Source: three-view drawing plus pictorial views. Frame: mm from the lowest corner of the part. A direction names the side the tool comes from. Coordinates: 2 decimals unless noted, no trailing zeros. Write each loop counter-clockwise with the first axis right and the second up, starting at its lowest first coordinate (ties: lowest second). Pieces come first, ordered by that corner, then holes. Notation, with made-up numbers: M -15.5,64 L 36.5,64 A28 ccw 36.5,98 Z; hole C 18.25,30.25 d3. An arc over 180 degrees is marked long. Write item = value, one per line. Start each with the question number.
Item 1: Section B-B on y = 20. Output: boundary loops of the cut face in (x, z), plus the area to 3 significant figures.
Item 2: Section A-A on x = 27.5. Output: boundary loops of the cut face in (y, z).
Item 3: Section D-D on z = 12. Output: boundary loops of the cut face in (x, y).
Item 4: Ray query, L1, parallel to X at y = 4.5, z = 15.5; L2, parallel to Y at x = 15, z = 26; L3, parallel to X at y = 16.5, z = 40. Return the intervals inside material, ascending. Write a range as [from, to].
Item 5: First-contact query: pin 1 Ø15 at (y, z) = (32.5, 38) entering from +X; pin 2 Ø13.5 at (x, z) = (19, 28) entering from -Y; pin 3 Ø8 at (x, y) = (78.5, 4) entering from +Z. Flat tips, straight axial feed; report the tip coordinate or a pass-through.
Item 6: Pull-direction query (X, two-part tool) for the marked faces 6, 7 and 8; classes: +X half, -X half, draft (parallel to the pull), parting line (faces both ways), or undercut.
Item 7: Reachability of the marked faces 1, 2, 3, 4 and 5 from +Z, -Z, +X, -X, +Y, -Y: full face, straight path, thin tool, end or side. Return the list, or none.
Item 8: Section C-C on z = 41.5. Output: boundary loops of the cut face in (x, y), plus the area to 4 significant figures.
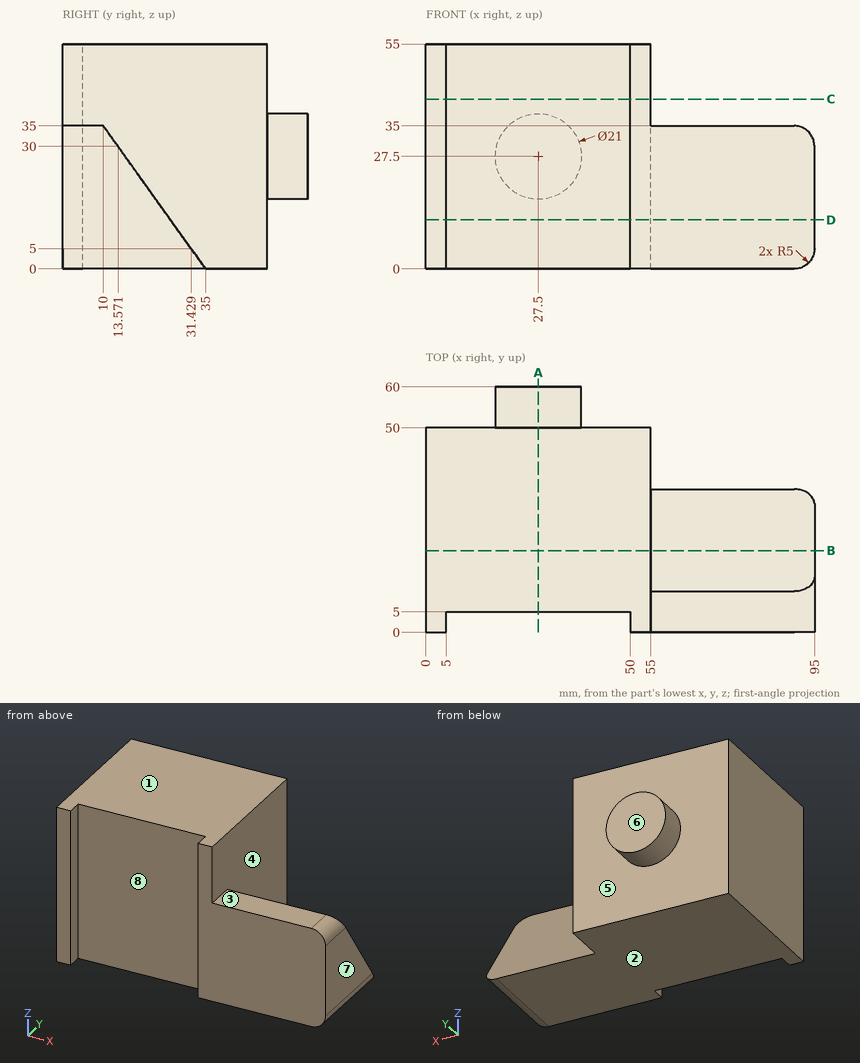
Responses:
q1.outline = M 0,0 L 90,0 A5 ccw 95,5 L 95,21 L 55,21 L 55,55 L 0,55 Z
q1.area = 3,860 mm²
q2.outline = M 5,0 L 50,0 L 50,17 L 60,17 L 60,38 L 50,38 L 50,55 L 5,55 Z
q3.outline = M 0,0 L 5,0 L 5,5 L 50,5 L 50,0 L 95,0 L 95,26.43 L 55,26.43 L 55,50 L 0,50 Z
q4.L1 = [0, 5], [50, 95]
q4.L2 = [5, 50]
q4.L3 = [0, 55]
q5.pin_1 = 55
q5.pin_2 = 5
q5.pin_3 = 35
q6.face_6 = draft
q6.face_7 = +X half
q6.face_8 = undercut
q7.face_1 = +Z, +X, -X, +Y, -Y
q7.face_2 = -Z, +X, -X, +Y, -Y
q7.face_3 = +Z, +X, +Y, -Y
q7.face_4 = +Z, +X, +Y
q7.face_5 = +Y
q8.outline = M 0,0 L 5,0 L 5,5 L 50,5 L 50,0 L 55,0 L 55,50 L 0,50 Z
q8.area = 2,525 mm²
